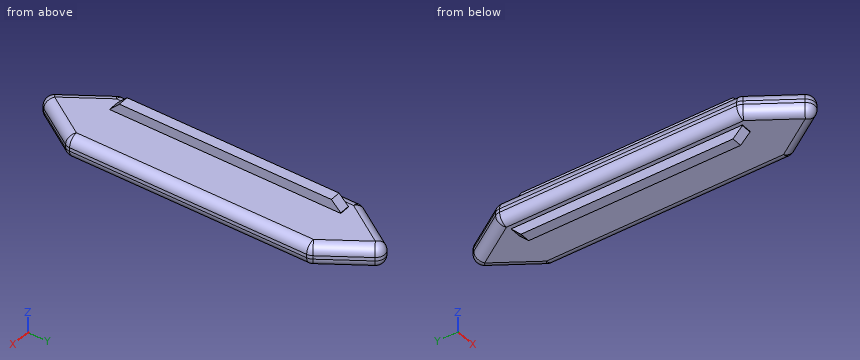
from build123d import *

# Parameters (mm, degrees)
F0_W     = 2.225
F0_H     = 49.06
F1_DEPTH = 4.5
F2_DEPTH = 2.375
F3_R     = 2
F4_SIZE  = 2


with BuildPart() as f1:
    # F0 (on Top) → F1 (new body, symmetric)
    with BuildSketch(Plane.XY):
        with Locations((-3.8675, 37.93)):
            Rectangle(F0_W, F0_H)
    extrude(amount=F1_DEPTH, both=True)

    # F0 (on Top) → F2 (join, symmetric)
    with BuildSketch(Plane.XY):
        Polygon((-7.84, 11.935359), (0, 0), (7.84, 11.935359), (7.84, 63.524641), (0, 75.46), (-7.84, 63.524641), align=None)
        with Locations((-3.8675, 37.93)):
            Rectangle(F0_W, F0_H, mode=Mode.SUBTRACT)
    extrude(amount=F2_DEPTH, both=True)

    # F3
    f3_edges = [f1.edges().sort_by_distance(p)[0] for p in [
        (-7.84, 37.73, 2.375),
        (-3.92, 69.49232, 2.375),
        (3.92, 69.49232, 2.375),
        (7.84, 37.73, 2.375),
        (-3.92, 5.96768, 2.375),
        (3.92, 5.96768, 2.375),
        (-3.92, 5.96768, -2.375),
        (-7.84, 37.73, -2.375),
        (3.92, 5.96768, -2.375),
        (7.84, 37.73, -2.375),
        (3.92, 69.49232, -2.375),
        (-3.92, 69.49232, -2.375),
        (0, 75.46, 0),
        (-7.84, 63.524641, 0),
        (7.84, 63.524641, 0),
        (7.84, 11.935359, 0),
        (-7.84, 11.935359, 0),
        (0, 0, 0),
    ]]
    fillet(f3_edges, radius=F3_R)

    # F4
    f4_edges = [f1.edges().sort_by_distance(p)[0] for p in [
        (-3.8675, 62.46, 4.5),
        (-3.8675, 62.46, -4.5),
        (-3.8675, 13.4, 4.5),
        (-3.8675, 13.4, -4.5),
    ]]
    chamfer(f4_edges, length=F4_SIZE)


solid = f1.part
The model under review builds one solid part; all positions refer to its coordinate system, in mm. Round coordinates to 2 decimals unless told otherwise and drop trailing zeros. Write each loop counter-clockwise with the first axis right and the second up, starting at its lowest first coordinate (ties: lowest second). Pieces come first, ordered by that corner, then holes. Notation, with made-up numbers: M 71,12 L 112,12 A12 ccw 112,35 Z; hole C 28.25,35 d2. An arc over 180 degrees is marked long. Answer as CSV lines item,"result". Start each with the question number.
Q1. Wall thickness on line 1 along X through (y, z) = (27, 3) (3 decimals); line 2 along X through (y, z) = (19, 0.5); line 3 along Z through (x, y) = (3.5, 14) (3 decimals): over which ranges is each line inside the solid? List them lowest first.
Q2. Consider section B-B, the plane z = -1.75. Give the boundary of the cut face in (x, y).
Q3. Consider section C-C, the plane z = 1.5. Give the boundary of the cut face in (x, y) (3 decimals), then the cut area to 3 significant figures.
Q4. Clearance check with flat-ended pins moving along their axes: P1, Ø0.6, axis at y = 47, z = -3, coming from the -X side; P2, Ø1.7, axis at y = 39, z = -3.5, coming from the +X side (3 decimals); P3, Ø3, axis at x = 1, y = 29.5, coming from the +Z side (3 decimals). State where each tip first meets the part, or that it passes through.
Q5. Consider section A-A, the plane y = 57.5. Give the boundary of the cut face in (x, z) (3 decimals).
Result set:
1,line 1,"x = -4.98 to -2.755"
1,line 2,"x = -7.84 to 7.84"
1,line 3,"z = -2.375 to 2.375"
2,outline,"M -7.29,12.53 A1.45 ccw -7.05,11.74 L -1.21,2.85 A1.45 ccw 1.21,2.85 L 7.05,11.74 A1.45 ccw 7.29,12.53 L 7.29,62.93 A1.45 ccw 7.05,63.72 L 1.21,72.61 A1.45 ccw -1.21,72.61 L -7.05,63.72 A1.45 ccw -7.29,62.93 Z"
3,outline,"M -7.494,12.533 A1.654 ccw -7.222,11.626 L -1.382,2.735 A1.654 ccw 1.382,2.735 L 7.222,11.626 A1.654 ccw 7.494,12.533 L 7.494,62.927 A1.654 ccw 7.222,63.834 L 1.382,72.725 A1.654 ccw -1.382,72.725 L -7.222,63.834 A1.654 ccw -7.494,62.927 Z"
3,area,"938 mm²"
4,P1,"stops at x = -4.98"
4,P2,"stops at x = -2.755"
4,P3,"stops at z = 2.375"
5,outline,"M -7.84,-0.375 A2 ccw -5.84,-2.375 L -4.98,-2.375 L -4.98,-4.5 L -2.755,-4.5 L -2.755,-2.375 L 5.84,-2.375 A2 ccw 7.84,-0.375 L 7.84,0.375 A2 ccw 5.84,2.375 L -2.755,2.375 L -2.755,4.5 L -4.98,4.5 L -4.98,2.375 L -5.84,2.375 A2 ccw -7.84,0.375 Z"
